Check sheet for the modelled part. Datum: model origin and axes. Units: mm. A direction names the side the tool comes from. Round coordinates to 2 decimals unless told otherwise and drop trailing zeros. Write each loop counter-clockwise with the first axis right and the second up, starting at its lowest first coordinate (ties: lowest second). Pieces come first, ordered by that corner, then holes.
Item 1: Release check for a two-part mould opening along Y. For faces 6 (the cylindrical face through (0, 29, -12)), 7 (the flat face through (0, 12, 5)), 8 (the cylindrical face through (-3, 0, 1)) record: pulls with the +Y half, pulls with the -Y half, needs draft (parallel to the pull), parting line crosses it, or undercut.
Item 2: Set-up check for faces 1 (the flat face through (0, 35, -15)), 2 (the flat face through (-0.1, -3.3, 3)), 3 (the flat face through (0, 47, -5)), 4 (the flat face through (0, 41.75, -8)), 5 (the flat face through (0, 21, -10)): record each of +Z, -Z, +X, -X, +Y, -Y from which the full face is reachable in a straight line by a thin tool's end or side.
Item 3: Section check C-C, the plane y = 23. Record the cut outline in (x, z).
Item 4: Material ranges on line 1 along X through (y, z) = (0, 3.05); line 2 along X through (y, z) = (0, 2.5); line 3 along Y through (x, z) = (9, -7.25), recorded low to high.
Item 5: Depth check by flat-ended pin: pin 1 (3 mm diameter, centred on x = 1.5, y = -0.5, fed in from +Z); pin 2 (2 mm diameter, centred on y = -2.5, z = 0, fed in from -X); pin 3 (8 mm diameter, centred on x = 0, y = 0, fed in from -Z); pin 4 (7 mm diameter, centred on x = -7, y = 37, fed in from -Z). Enter the tip coordinate at first touch or a pass-through.
Item 6: Section check D-D, the plane z = 1.25. Record the cut outline in (x, y).
Item 7: Section check B-B, the plane z = -8.5. Record the cut outline in (x, y), plus the area to 3 significant figures.
from build123d import *

# Parameters (mm, degrees)
ESBO_O2_R                = 3
RESSALTO_EXTRUS_O1_DEPTH = 5
ESBO_O7_R                = 5
CORTE_EXTRUS_O2_DEPTH    = 2
ESBO_O3_W                = 45
ESBO_O3_H                = 13
RESSALTO_EXTRUS_O2_DEPTH = 10
ESBO_O4_W                = 45
ESBO_O4_H                = 20
RESSALTO_EXTRUS_O3_DEPTH = 17
ESBO_O6_W                = 30.5
ESBO_O6_H                = 6.5
CORTE_EXTRUS_O1_DEPTH    = 15
FILETE4_R                = 5
FILETE5_R                = 2


with BuildPart() as part:
    # Esboço2 → Ressalto-extrusão1 (new body)
    with BuildSketch(Plane.XY):
        with BuildLine():
            Line((-22.5, 0), (-22.5, 30))
            Line((-22.5, 30), (22.5, 30))
            Line((22.5, 30), (22.5, 0))
            ThreePointArc((22.5, 0), (0, -22.5), (-22.5, 0))
        make_face()
        Circle(ESBO_O2_R, mode=Mode.SUBTRACT)
    extrude(amount=RESSALTO_EXTRUS_O1_DEPTH)

    # Esboço7 → Corte-extrusão2 (cut)
    with BuildSketch(Plane.XY.offset(5)):
        Circle(ESBO_O7_R)
    extrude(amount=-CORTE_EXTRUS_O2_DEPTH, mode=Mode.SUBTRACT)

    # Esboço3 → Ressalto-extrusão2 (add)
    with BuildSketch(Plane(origin=(0, 0, 0), x_dir=(-1, 0, 0), z_dir=(0, 0, -1))):
        with Locations((0, 23.5)):
            Rectangle(ESBO_O3_W, ESBO_O3_H)
    extrude(amount=RESSALTO_EXTRUS_O2_DEPTH)

    # Esboço4 → Ressalto-extrusão3 (add)
    with BuildSketch(Plane(origin=(0, 30, 0), x_dir=(1, 0, 0), z_dir=(0, 1, 0))):
        with Locations((0, 5)):
            Rectangle(ESBO_O4_W, ESBO_O4_H)
    extrude(amount=RESSALTO_EXTRUS_O3_DEPTH)

    # Esboço6 → Corte-extrusão1 (cut)
    with BuildSketch(Plane(origin=(0, 0, -15), x_dir=(-1, 0, 0), z_dir=(0, 0, -1))):
        with Locations((0, 38.5)):
            Rectangle(ESBO_O6_W, ESBO_O6_H)
    extrude(amount=-CORTE_EXTRUS_O1_DEPTH, mode=Mode.SUBTRACT)

    # Filete4
    filete4_edges = [part.edges().sort_by_distance(p)[0] for p in [
        (0, 30, -10),
    ]]
    fillet(filete4_edges, radius=FILETE4_R - 0.0001)  # a hair under: the kernel refuses the full size

    # Filete5
    filete5_edges = [part.edges().sort_by_distance(p)[0] for p in [
        (-5, 0, 5),
    ]]
    fillet(filete5_edges, radius=FILETE5_R - 0.0001)  # a hair under: the kernel refuses the full size


solid = part.part
Values found:
1. face 6: pulls with the -Y half
1. face 7: needs draft
1. face 8: undercut
2. face 1: -Z, +X, -X, +Y, -Y
2. face 2: +Z
2. face 3: +Z, -Z, +X, -X, +Y
2. face 4: -Z
2. face 5: -Z, +X, -X, -Y
3. outline: (-22.5, -10) - (22.5, -10) - (22.5, 5) - (-22.5, 5) - close
4. line 1: x = -22.5 to -5, 5 to 22.5
4. line 2: x = -22.5 to -3, 3 to 22.5
4. line 3: y = 17 to 35.25, 41.75 to 47
5. pin 1: stops at z = 3
5. pin 2: stops at x = -22.45
5. pin 3: stops at z = 0
5. pin 4: stops at z = -15
6. outline: (-22.5, 0) arc R22.5 ccw to (22.5, 0) - (22.5, 47) - (-22.5, 47) - close; hole circle Ø6 at (0, 0)
7. outline: (-22.5, 17) - (22.5, 17) - (22.5, 47) - (-22.5, 47) - close; hole (-15.25, 35.25) - (15.25, 35.25) - (15.25, 41.75) - (-15.25, 41.75) - close
7. area: 1,150 mm2
